Here's how the part is built. I have some questions about the finished solid (model axes, mm). A direction names the side the tool comes from. Give positions to 0.01 mm unless a question says otherwise; leave off trailing zeros. Loops run counter-clockwise (first coordinate to the right, second up) from the corner with the lowest first, then second, coordinate; pieces in that order, holes last. Notation, with made-up numbers: (48.5, 18) - (62.5, 18) arc R8 ccw to (62.5, 24) - close; hole circle Ø4 at (-24, 30.5). An arc over 180 degrees is marked (long way). Return JSON: item names as keys, results as strings. Group by question number.
(1) I need wall thicknesses on probe 1 along X at (y, z) = (-2, 0); probe 2 along X at (y, z) = (1, 0); probe 3 along Y at (x, z) = (-5, 18) (3 decimals). Which ranges of each line are inside material? Lowest first, please. Write a range as [from, to].
(2) If we mould it in two halves opening along Z, with no side actions, what happens to faces 6 (the cylindrical face through (3.92, -1.6, -14.21)), 7 (the cylindrical face through (12.88, -4.8, 11.79)), 8 (the cylindrical face through (-2.41, -1.55, -10.85))? For each: released by +Z, released by -Z, zero draft, split by the parting line, or undercut.
(3) For P1, Ø0.6, axis at x = 0.5, z = 11.5, coming from the +Y side; P2, Ø20, axis at x = 0, z = 0, coming from the -Y side; P3, Ø2, axis at y = 2.5, z = 12, coming from the +X side, each with a flat end and sliding along its axis, tell me the tip position at first contact or that it passes through.
(4) On a 3-axis mill with a long thin cutter (end or side, diameter ignored), from which of +Z, -Z, +X, -X, +Y, -Y can I reach the whole of each face in a straight line? I mean faces 1 (the cylindrical face through (-6.984, -4.804, 12.955)), 2 (the cylindrical face through (7.727, -4.804, 12.526)), 3 (the cylindrical face through (0.88, -3.162, 14.716)), 4 (the flat face through (5, -3.238, -15)), 5 (the cylindrical face through (-0.88, -3.162, -14.716)). Say none if no direction works.
(5) If we section it at A-A (y = 2): Please give me the cut outline in (x, z) (1 decimal), then the cut area to 3 significant figures.
```python
from build123d import *

# Parameters (mm, degrees)
SKETCH1_W           = 50.8
SKETCH1_H           = 50.8
SKETCH1_R           = 11.1125
BOSS_EXTRUDE1_DEPTH = 3.175
SKETCH2_R           = 11.1125
BOSS_EXTRUDE2_DEPTH = 3.2385
SKETCH3_R           = 11.1125
BOSS_EXTRUDE3_DEPTH = 3.175
SKETCH4_W           = 3.81
SKETCH4_H           = 1.905
CUT_EXTRUDE1_DEPTH  = 1.905
CUT_EXTRUDE2_DEPTH  = 4.175


with BuildPart() as part:
    # Sketch1 → Boss-Extrude1 (new body)
    with BuildSketch(Plane(origin=(0, 0, 0), x_dir=(1, 0, 0), z_dir=(0, 1, 0))):
        Rectangle(SKETCH1_W, SKETCH1_H)
        Circle(SKETCH1_R, mode=Mode.SUBTRACT)
    extrude(amount=BOSS_EXTRUDE1_DEPTH)

    # Sketch2 → Boss-Extrude2 (add)
    with BuildSketch(Plane.XZ):
        with BuildLine():
            ThreePointArc((-14.076948351, 2.368425674), (-14.196601152, -1.492122907), (-13.276909868, -5.243432024))
            ThreePointArc((-13.276909868, -5.243432024), (-13.179807483, -6.577553377), (-13.860975695, -7.72877817))
            ThreePointArc((-13.860975695, -7.72877817), (-14.480846101, -8.94534234), (-14.127459264, -10.264199968))
            ThreePointArc((-14.127459264, -10.264199968), (-12.982353661, -11.007840242), (-11.63378189, -10.794247457))
            ThreePointArc((-11.63378189, -10.794247457), (-10.328409495, -10.502166015), (-9.089590976, -11.006782042))
            ThreePointArc((-9.089590976, -11.006782042), (-5.806084233, -13.040678699), (-2.097509598, -14.119857242))
            ThreePointArc((-2.097509598, -14.119857242), (-0.893575422, -14.702824786), (-0.237169612, -15.868346158))
            ThreePointArc((-0.237169612, -15.868346158), (0.506470662, -17.013451761), (1.82532829, -17.366838598))
            ThreePointArc((1.82532829, -17.366838598), (3.04189246, -16.746968192), (3.531201567, -15.472274387))
            ThreePointArc((3.531201567, -15.472274387), (3.930937816, -14.195748011), (4.987357374, -13.375207717))
            ThreePointArc((4.987357374, -13.375207717), (8.390516919, -11.548555791), (11.17940027, -8.876425218))
            ThreePointArc((11.17940027, -8.876425218), (12.286232061, -8.125271409), (13.623806083, -8.139567988))
            ThreePointArc((13.623806083, -8.139567988), (14.987316762, -8.068109421), (15.952787554, -7.10263863))
            ThreePointArc((15.952787554, -7.10263863), (16.024246121, -5.73912795), (15.164983457, -4.67802693))
            ThreePointArc((15.164983457, -4.67802693), (14.259347311, -3.693581996), (14.076948351, -2.368425674))
            ThreePointArc((14.076948351, -2.368425674), (14.196601152, 1.492122907), (13.276909868, 5.243432024))
            ThreePointArc((13.276909868, 5.243432024), (13.179807483, 6.577553377), (13.860975695, 7.72877817))
            ThreePointArc((13.860975695, 7.72877817), (14.480846101, 8.94534234), (14.127459264, 10.264199968))
            ThreePointArc((14.127459264, 10.264199968), (12.982353661, 11.007840242), (11.63378189, 10.794247457))
            ThreePointArc((11.63378189, 10.794247457), (10.328409495, 10.502166015), (9.089590976, 11.006782042))
            ThreePointArc((9.089590976, 11.006782042), (5.806084233, 13.040678699), (2.097509598, 14.119857242))
            ThreePointArc((2.097509598, 14.119857242), (0.893575422, 14.702824786), (0.237169612, 15.868346158))
            ThreePointArc((0.237169612, 15.868346158), (-0.506470662, 17.013451761), (-1.82532829, 17.366838598))
            ThreePointArc((-1.82532829, 17.366838598), (-3.04189246, 16.746968192), (-3.531201567, 15.472274387))
            ThreePointArc((-3.531201567, 15.472274387), (-3.930937816, 14.195748011), (-4.987357374, 13.375207717))
            ThreePointArc((-4.987357374, 13.375207717), (-8.390516919, 11.548555791), (-11.17940027, 8.876425218))
            ThreePointArc((-11.17940027, 8.876425218), (-12.286232061, 8.125271409), (-13.623806083, 8.139567988))
            ThreePointArc((-13.623806083, 8.139567988), (-14.987316762, 8.068109421), (-15.952787554, 7.10263863))
            ThreePointArc((-15.952787554, 7.10263863), (-16.024246121, 5.73912795), (-15.164983457, 4.67802693))
            ThreePointArc((-15.164983457, 4.67802693), (-14.259347311, 3.693581996), (-14.076948351, 2.368425674))
        make_face()
        Circle(SKETCH2_R, mode=Mode.SUBTRACT)
    extrude(amount=BOSS_EXTRUDE2_DEPTH)

    # Sketch3 → Boss-Extrude3 (add)
    with BuildSketch(Plane.XZ.offset(3.2385)):
        with BuildLine():
            ThreePointArc((-13.623806083, 8.139567988), (-12.286232061, 8.125271409), (-11.17940027, 8.876425218))
            ThreePointArc((-11.17940027, 8.876425218), (-9.625048397, 10.541743612), (-7.82558077, 11.938601285))
            ThreePointArc((-7.82558077, 11.938601285), (-6.977108558, 12.97272099), (-6.869996245, 14.30607601))
            ThreePointArc((-6.869996245, 14.30607601), (-6.675129359, 15.657480685), (-5.626048811, 16.531378679))
            ThreePointArc((-5.626048811, 16.531378679), (-3.749033675, 17.05531157), (-1.82532829, 17.366838598))
            ThreePointArc((-1.82532829, 17.366838598), (-0.506470662, 17.013451761), (0.237169612, 15.868346158))
            ThreePointArc((0.237169612, 15.868346158), (0.893575422, 14.702824786), (2.097509598, 14.119857242))
            ThreePointArc((2.097509598, 14.119857242), (4.31689357, 13.606408231), (6.426341614, 12.746452389))
            ThreePointArc((6.426341614, 12.746452389), (7.746151654, 12.528713751), (8.954427131, 13.102629278))
            ThreePointArc((8.954427131, 13.102629278), (10.222211353, 13.609571941), (11.50356949, 13.137990533))
            ThreePointArc((11.50356949, 13.137990533), (12.895816252, 11.774414187), (14.127459264, 10.264199968))
            ThreePointArc((14.127459264, 10.264199968), (14.480846101, 8.94534234), (13.860975695, 7.72877817))
            ThreePointArc((13.860975695, 7.72877817), (13.179807483, 6.577553377), (13.276909868, 5.243432024))
            ThreePointArc((13.276909868, 5.243432024), (13.941941967, 3.064664618), (14.251922384, 0.807851103))
            ThreePointArc((14.251922384, 0.807851103), (14.723260212, -0.444007239), (15.824423376, -1.203446733))
            ThreePointArc((15.824423376, -1.203446733), (16.897340712, -2.047908744), (17.129618301, -3.393388146))
            ThreePointArc((17.129618301, -3.393388146), (16.644849927, -5.280897383), (15.952787554, -7.10263863))
            ThreePointArc((15.952787554, -7.10263863), (14.987316762, -8.068109421), (13.623806083, -8.139567988))
            ThreePointArc((13.623806083, -8.139567988), (12.286232061, -8.125271409), (11.17940027, -8.876425218))
            ThreePointArc((11.17940027, -8.876425218), (9.625048397, -10.541743612), (7.82558077, -11.938601285))
            ThreePointArc((7.82558077, -11.938601285), (6.977108558, -12.97272099), (6.869996245, -14.30607601))
            ThreePointArc((6.869996245, -14.30607601), (6.675129359, -15.657480685), (5.626048811, -16.531378679))
            ThreePointArc((5.626048811, -16.531378679), (3.749033675, -17.05531157), (1.82532829, -17.366838598))
            ThreePointArc((1.82532829, -17.366838598), (0.506470662, -17.013451761), (-0.237169612, -15.868346158))
            ThreePointArc((-0.237169612, -15.868346158), (-0.893575422, -14.702824786), (-2.097509598, -14.119857242))
            ThreePointArc((-2.097509598, -14.119857242), (-4.31689357, -13.606408231), (-6.426341614, -12.746452389))
            ThreePointArc((-6.426341614, -12.746452389), (-7.746151654, -12.528713751), (-8.954427131, -13.102629278))
            ThreePointArc((-8.954427131, -13.102629278), (-10.222211353, -13.609571941), (-11.50356949, -13.137990533))
            ThreePointArc((-11.50356949, -13.137990533), (-12.895816252, -11.774414187), (-14.127459264, -10.264199968))
            ThreePointArc((-14.127459264, -10.264199968), (-14.480846101, -8.94534234), (-13.860975695, -7.72877817))
            ThreePointArc((-13.860975695, -7.72877817), (-13.179807483, -6.577553377), (-13.276909868, -5.243432024))
            ThreePointArc((-13.276909868, -5.243432024), (-13.941941967, -3.064664618), (-14.251922384, -0.807851103))
            ThreePointArc((-14.251922384, -0.807851103), (-14.723260212, 0.444007239), (-15.824423376, 1.203446733))
            ThreePointArc((-15.824423376, 1.203446733), (-16.897340712, 2.047908744), (-17.129618301, 3.393388146))
            ThreePointArc((-17.129618301, 3.393388146), (-16.644849927, 5.280897383), (-15.952787554, 7.10263863))
            ThreePointArc((-15.952787554, 7.10263863), (-14.987316762, 8.068109421), (-13.623806083, 8.139567988))
        make_face()
        Circle(SKETCH3_R, mode=Mode.SUBTRACT)
    extrude(amount=BOSS_EXTRUDE3_DEPTH)

    # Sketch4 → Cut-Extrude1 (cut)
    with BuildSketch(Plane(origin=(0, 3.175, 0), x_dir=(1, 0, 0), z_dir=(0, 1, 0))):
        with Locations((0, -11.900496677)):
            Rectangle(SKETCH4_W, SKETCH4_H)
    extrude(amount=-CUT_EXTRUDE1_DEPTH, mode=Mode.SUBTRACT)

    # Sketch5 → Cut-Extrude2 (cut, through all)
    with BuildSketch(Plane.XZ):
        with BuildLine():
            Line((20.423083051, 25.4), (24.80772592, 5.45313989))
            ThreePointArc((24.80772592, 5.45313989), (25.251497365, 2.74260475), (25.4, 0))
            Line((25.4, 0), (25.4, 25.4))
            Line((25.4, 25.4), (20.423083051, 25.4))
        make_face()
    extrude(amount=-CUT_EXTRUDE2_DEPTH, mode=Mode.SUBTRACT)


solid = part.part
```
Values:
{
 "1": {"probe 1": "[-14.27, -11.11], [11.11, 14.27]", "probe 2": "[-25.4, -11.11], [11.11, 25.4]", "probe 3": "[0, 3.175]"},
 "2": {"face 6": "released by -Z", "face 7": "released by +Z", "face 8": "undercut"},
 "3": {"P1": "y = 1.27", "P2": "through", "P3": "x = 23.59"},
 "4": {"face 1": "-X, -Y", "face 2": "+Z, -Y", "face 3": "+Z, +X, -Y", "face 4": "-Z, +X", "face 5": "-Z, -X, -Y"},
 "5": {"outline": "(-25.4, -25.4) - (25.4, -25.4) - (25.4, 0) arc R25.4 ccw to (24.8, 5.5) - (20.4, 25.4) - (-25.4, 25.4) - close; hole (-1.9, 10.9) arc R11.1 ccw (long way) to (1.9, 10.9) - (1.9, 12.9) - (-1.9, 12.9) - close", "area": "2,130 mm2"}
}
